Verification items for the finished model (mm, model axes). Face numbers are marked on the shaded views. A direction names the side the tool comes from. Coordinates: 2 decimals unless noted, no trailing zeros. Loops run counter-clockwise (first coordinate to the right, second up) from the corner with the lowest first, then second, coordinate; pieces in that order, holes last. Notation, with made-up numbers: (78.5, 85) - (117.5, 85) arc R15 cw to (117.5, 103) - close; hole circle Ø2 at (0, 53). An arc over 180 degrees is marked (long way). One line per item, written item: value. Start each with the question number.
(1) Section check A-A (z = 16). Record the boundary of the cut face in (x, y).
(2) Gauge pin test, flat ends, axial feed: P1, Ø7.5, axis at y = 282, z = 14, coming from the +X side; P2, Ø18, axis at x = 320.5, y = 302, coming from the +Z side; P3, Ø5.5, axis at x = 327, z = 8, coming from the +Y side. Record the tip position at first contact, or that the pin passes through.
(3) Section check C-C (x = 317). Record the boundary of the cut face in (y, z).
(4) Thickness scan on probe 1 along Y at (x, z) = (329.3, 17); probe 2 along Z at (x, y) = (312, 284); probe 3 along X at (y, z) = (285, 9.5). Record the ranges inside material, lowest first. Write a range as [from, to].
(5) Section check B-B (z = 13.25). Record the boundary of the cut face in (x, y), plus the area to 3 significant figures.
(6) Set-up check for the marked faces 1, 2 and 3: record each of +Z, -Z, +X, -X, +Y, -Y from which the full face is reachable in a straight line by a thin tool's end or side.
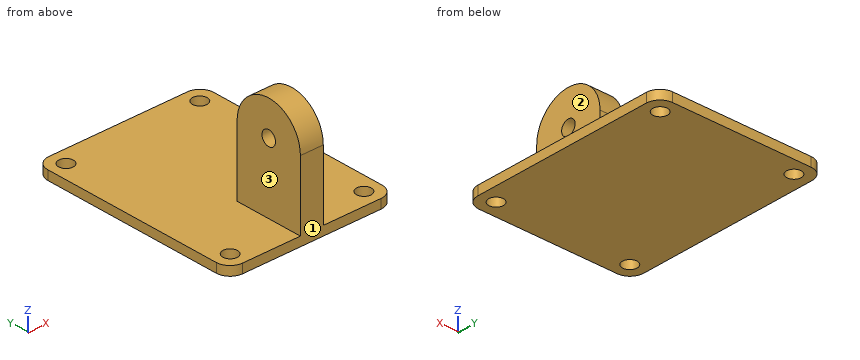
```python
from build123d import *

# Parameters (mm, degrees)
MODEL_R             = 1.6
EXTRUDE_1_DEPTH     = 2
SKETCH_2_W          = 5
SKETCH_2_H          = 15
EXTRUDE_2_DEPTH     = 15
EXTRUDE_3_DEPTH     = 5
SKETCH_4_R          = 1.6
CUT_EXTRUDE_1_DEPTH = 5


with BuildPart() as part:
    # Model → 凸台-拉伸1 (new body)
    with BuildSketch(Plane.XY):
        with BuildLine():
            Line((312.88241623, 324.041107056), (343.08241623, 324.041107056))
            ThreePointArc((343.08241623, 324.041107056), (345.203736573, 323.1624274), (346.08241623, 321.041107056))
            Line((346.08241623, 321.041107056), (346.08241623, 281.141107056))
            ThreePointArc((346.08241623, 281.141107056), (345.203736573, 279.019786713), (343.08241623, 278.141107056))
            Line((343.08241623, 278.141107056), (312.88241623, 278.141107056))
            ThreePointArc((312.88241623, 278.141107056), (310.761095886, 279.019786713), (309.88241623, 281.141107056))
            Line((309.88241623, 281.141107056), (309.88241623, 321.041107056))
            ThreePointArc((309.88241623, 321.041107056), (310.761095886, 323.1624274), (312.88241623, 324.041107056))
        make_face()
        with Locations((313.38241623, 320.541107056)):
            Circle(MODEL_R, mode=Mode.SUBTRACT)
        with Locations((313.38241623, 281.641107056)):
            Circle(MODEL_R, mode=Mode.SUBTRACT)
        with Locations((342.58241623, 320.541107056)):
            Circle(MODEL_R, mode=Mode.SUBTRACT)
        with Locations((342.58241623, 281.641107056)):
            Circle(MODEL_R, mode=Mode.SUBTRACT)
    extrude(amount=EXTRUDE_1_DEPTH)

    # 草图2 → 凸台-拉伸2 (add)
    with BuildSketch(Plane.XY.offset(2)):
        with Locations((327.98241623, 285.641107056)):
            Rectangle(SKETCH_2_W, SKETCH_2_H)
    extrude(amount=EXTRUDE_2_DEPTH)

    # 草图3 → 凸台-拉伸3 (add)
    with BuildSketch(Plane.ZY.offset(-325.48241623)):
        with BuildLine():
            Line((17, 293.141107056), (17, 278.141107056))
            ThreePointArc((17, 278.141107056), (24.5, 285.641107056), (17, 293.141107056))
        make_face()
    extrude(amount=-EXTRUDE_3_DEPTH)

    # 草图4 → 切除-拉伸1 (cut)
    with BuildSketch(Plane.ZY.offset(-325.48241623)):
        with Locations((17, 285.641107056)):
            Circle(SKETCH_4_R)
    extrude(amount=-CUT_EXTRUDE_1_DEPTH, mode=Mode.SUBTRACT)


solid = part.part
```
Responses:
1. outline: (325.48, 278.14) - (330.48, 278.14) - (330.48, 284.39) - (325.48, 284.39) - close; (325.48, 286.89) - (330.48, 286.89) - (330.48, 293.14) - (325.48, 293.14) - close
2. P1: stops at x = 330.48
2. P2: stops at z = 2
2. P3: stops at y = 293.14
3. outline: (278.14, 0) - (324.04, 0) - (324.04, 2) - (278.14, 2) - close
4. probe 1: y = [278.14, 284.04], [287.24, 293.14]
4. probe 2: z = [0, 2]
4. probe 3: x = [325.48, 330.48]
5. outline: (325.48, 278.14) - (330.48, 278.14) - (330.48, 293.14) - (325.48, 293.14) - close
5. area: 75.0 mm²
6. face 1: +Z, -Z, +X, -X, -Y
6. face 2: +Z, +X, +Y, -Y
6. face 3: +Z, -X, +Y, -Y
